```python
from build123d import *

# Parameters (mm, degrees)
F0_W     = 68
F0_H     = 9.175
F0_R     = 1.5
F1_DEPTH = 3.175


# Not quite as in the source:
# - a length typed as a fraction of an inch, garbled in the dataset ("3 / 203.2 mm" for 3/8 in), is restored


with BuildPart() as f1:
    # F0 (on Top) → F1 (new body)
    with BuildSketch(Plane.XY):
        with Locations((28.9220271409, 16.632870598)):
            Rectangle(F0_W, F0_H)
        with Locations((-0.5779728591, 16.632870598)):
            Circle(F0_R, mode=Mode.SUBTRACT)
        Polygon((3.9220271409, 15.045370598), (3.9220271409, 18.220370598), (28.9220271409, 18.220370598), (53.9220271409, 18.220370598), (53.9220271409, 15.045370598), align=None, mode=Mode.SUBTRACT)
        with Locations((58.4220271409, 16.632870598)):
            Circle(F0_R, mode=Mode.SUBTRACT)
    extrude(amount=F1_DEPTH)


solid = f1.part
```
Geometry: final body of the model. Coordinates: model frame, mm. A direction names the side the tool comes from. Coordinates: 2 decimals unless noted, no trailing zeros. Order: outer loops, then holes, each group sorted by start corner. A loop starts at its lowest first (then second) coordinate and runs counter-clockwise, first axis right, second up. Notation, with made-up numbers: (45, 72.25) -> (53, 72.25) arc R34 ccw to (53, 111.25) -> close; hole circle Ø8 at (22, 85.25). An arc over 180 degrees is marked (long way). Write each question's results on one line, items separated by ' | '. Start each with the question number.
1) Cut plane A-A, the plane x = 42. Output: boundary loops of the cut face in (y, z) (3 decimals).
2) Set-up query: faces 1 (the flat face through (28, 19, 3.175)), 2 (the flat face through (53.922, 17, 2)). Return all of +Z, -Z, +X, -X, +Y, -Y with unobstructed straight access to the full face (end or side cutting, diameter ignored); none if empty.
3) Cut plane D-D, the plane x = -1. Output: boundary loops of the cut face in (y, z) (3 decimals), and give its area (3 significant figures).
4) Material intervals for line 1 along Y through (x, z) = (4, 1.35); line 2 along X through (y, z) = (17, 0.55); line 3 along X through (y, z) = (16, 1.25), sorted ascending.
5) Cut plane C-C, the plane z = 2. Output: boundary loops of the cut face in (x, y), and give its area (3 significant figures).
6) Mould query, pull axis X, two halves, no side actions, for faces 3 (the flat face through (-5.078, 17, 2)), 4 (the flat face through (29, 15.045, 2)), 5 (the flat face through (28, 19, 0)). Classes: released by +X, released by -X, zero draft, split by the parting line, or undercut.
7) Cut plane B-B, the plane y = 17.25. Output: boundary loops of the cut face in (x, z) (3 decimals).
Checks:
1) outline: (12.045, 0) -> (15.045, 0) -> (15.045, 3.175) -> (12.045, 3.175) -> close; (18.22, 0) -> (21.22, 0) -> (21.22, 3.175) -> (18.22, 3.175) -> close
2) face 1: +Z, +X, -X, +Y, -Y | face 2: +Z, -Z
3) outline: (12.045, 0) -> (15.193, 0) -> (15.193, 3.175) -> (12.045, 3.175) -> close; (18.072, 0) -> (21.22, 0) -> (21.22, 3.175) -> (18.072, 3.175) -> close | area: 20.0 mm^2
4) line 1: 12.05 to 15.05, 18.22 to 21.22 | line 2: -5.08 to -2.03, 0.88 to 3.92, 53.92 to 56.97, 59.88 to 62.92 | line 3: -5.08 to -1.94, 0.78 to 3.92, 53.92 to 57.06, 59.78 to 62.92
5) outline: (-5.08, 12.05) -> (62.92, 12.05) -> (62.92, 21.22) -> (-5.08, 21.22) -> close; hole circle Ø3 at (-0.58, 16.63); hole (3.92, 15.05) -> (53.92, 15.05) -> (53.92, 18.22) -> (3.92, 18.22) -> close; hole circle Ø3 at (58.42, 16.63) | area: 451 mm^2
6) face 3: released by -X | face 4: undercut | face 5: zero draft
7) outline: (-5.078, 0) -> (-1.945, 0) -> (-1.945, 3.175) -> (-5.078, 3.175) -> close; (0.789, 0) -> (3.922, 0) -> (3.922, 3.175) -> (0.789, 3.175) -> close; (53.922, 0) -> (57.055, 0) -> (57.055, 3.175) -> (53.922, 3.175) -> close; (59.789, 0) -> (62.922, 0) -> (62.922, 3.175) -> (59.789, 3.175) -> close
